Solid Edge part; units mm, degrees
sketch "Sketch1" plane through (0, 0, 0) normal (0, 0, 1) x (1, 0, 0)
  circle A0 centre (0, 0) radius 4.25
extrude "Protrusion1" add sketch "Sketch1" along normal blind 5
sketch "Sketch2" plane through (0, 0, 5) normal (0, 0, 1) x (1, 0, 0)
  circle A0 centre (0, 0) radius 2.5
extrude "ExtrudedProtrusion_2" add sketch "Sketch2" along normal blind 35
sketch "Sketch3" plane through (0, 0, 0) normal (0, 0, -1) x (-1, 0, 0)
  line L0 (2.25, 0) -> (1.125, 1.9486)
  line L1 (1.125, 1.9486) -> (-1.125, 1.9486)
  line L2 (-1.125, 1.9486) -> (-2.25, 0)
  line L3 (-2.25, 0) -> (-1.125, -1.9486)
  line L4 (-1.125, -1.9486) -> (1.125, -1.9486)
  line L5 (1.125, -1.9486) -> (2.25, 0)
extrude "ExtrudedCutout_1" cut sketch "Sketch3" against normal blind 2.6
cosmetic_thread "Thread_1" thread depth 24
properties material "Stainless steel"
Work out the finished part from the listing and answer in its coordinate system (mm). A direction names the side the tool comes from. Give positions to 0.01 mm unless a question says otherwise; leave off trailing zeros. Loops run counter-clockwise (first coordinate to the right, second up) from the corner with the lowest first, then second, coordinate; pieces in that order, holes last. Notation, with made-up numbers: (82, 12.25) - (106, 12.25) arc R16 cw to (106, 38.25) - close; hole circle Ø11 at (-33, -11). An arc over 180 degrees is marked (long way). Use CSV: the item, a comma, the result in double quotes. Start each with the question number.
(1) Find section B-B, the plane z = 22.5. Determine the outline of the cut face in (x, y), plus the area to 3 significant figures.
(2) Find the intervals of material crossed by L1, parallel to Z at x = 0, y = 1.75; L2, parallel to Z at x = 1, y = 3; L3, parallel to X at y = -1, z = 13, in increasing order.
(3) Determine the mould class of faces 1 (the face through (1.68, 0.99, 1.28)), 2 (the face through (0, 0, 40)), 3 (the face through (2.285, -3.584, 2.465)) for opening direction Y: released by +Y, released by -Y, zero draft, split by the parting line, or undercut.
(4) Find section C-C, the plane y = -1.5. Determine the outline of the cut face in (x, z).
(5) Each of these flat-tipped pins is pushed along its axis until it touches: pin 1 (3 mm diameter, centred on x = -2.5, y = 2, fed in from -Z); pin 2 (3 mm diameter, centred on y = 1.5, z = 23, fed in from +X); pin 3 (2 mm diameter, centred on y = -3, z = 12.5, fed in from +X); pin 4 (1.5 mm diameter, centred on x = 2, z = 6, fed in from +Y). Where does it stop, or does it pass through?
(6) Find section D-D, the plane x = -3.5. Determine the outline of the cut face in (y, z), plus the area to 3 significant figures.
(7) Find section A-A, the plane x = 0. Determine the outline of the cut face in (y, z), plus the area to 3 significant figures.
(8) A tool of negligible diameter and unlimited length cuts with its end or side. For faces 4 (the face through (2, -1, 0)), 5 (the face through (2, -2, 5)), 6 (the face through (1.695, -0.961, 1.282)), from which of +Z, -Z, +X, -X, +Y, -Y can it reach the whole face along a straight path? Write none if from no direction.
Results found:
1,outline,"circle Ø5 at (0, 0)"
1,area,"19.6 mm^2"
2,L1,"2.6 to 40"
2,L2,"0 to 5"
2,L3,"-2.29 to 2.29"
3,face 1,"undercut"
3,face 2,"zero draft"
3,face 3,"split by the parting line"
4,outline,"(-3.98, 0) - (-1.38, 0) - (-1.38, 2.6) - (1.38, 2.6) - (1.38, 0) - (3.98, 0) - (3.98, 5) - (2, 5) - (2, 40) - (-2, 40) - (-2, 5) - (-3.98, 5) - close"
5,pin 1,"z = 0"
5,pin 2,"x = 2.5"
5,pin 3,"x = 1.5"
5,pin 4,"y = 2.17"
6,outline,"(-2.41, 0) - (2.41, 0) - (2.41, 5) - (-2.41, 5) - close"
6,area,"24.1 mm^2"
7,outline,"(-4.25, 0) - (-1.95, 0) - (-1.95, 2.6) - (1.95, 2.6) - (1.95, 0) - (4.25, 0) - (4.25, 5) - (2.5, 5) - (2.5, 40) - (-2.5, 40) - (-2.5, 5) - (-4.25, 5) - close"
7,area,"207 mm^2"
8,face 4,"-Z, +X, -X, +Y, -Y"
8,face 5,"+Z"
8,face 6,"-Z"
